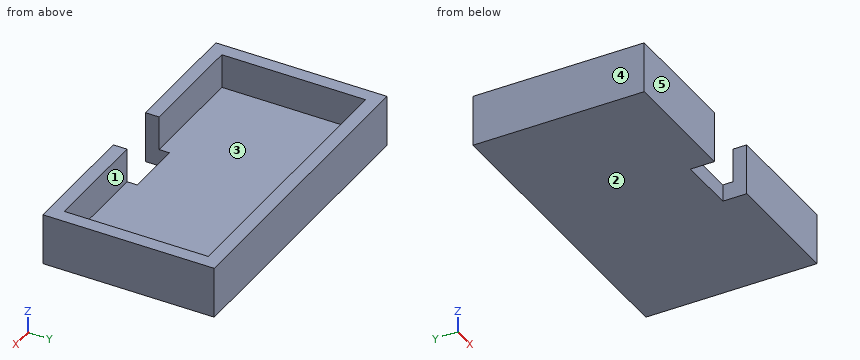
```python
from build123d import *

# Parameters (mm, degrees)
F0_W     = 57.15
F0_H     = 31.75
F1_DEPTH = 9.525
F2_W     = 52.07
F2_H     = 26.67
F3_DEPTH = 6.35
F4_W     = 10.668
F4_H     = 2.54
F4_H_2   = 1.905
F5_DEPTH = 25.4


with BuildPart() as f1:
    # F0 (on Top) → F1 (new body)
    with BuildSketch(Plane.XY):
        Rectangle(F0_W, F0_H)
    extrude(amount=F1_DEPTH)

    # F2 (on face) → F3 (cut)
    with BuildSketch(Plane.XY.offset(9.525)):
        Rectangle(F2_W, F2_H)
    extrude(amount=-F3_DEPTH, mode=Mode.SUBTRACT)

    # F4 (on face) → F5 (cut)
    with BuildSketch(Plane.XY.offset(9.525)):
        with Locations((0, -14.605)):
            Rectangle(F4_W, F4_H)
        with Locations((0, -12.3825)):
            Rectangle(F4_W, F4_H_2)
    extrude(amount=-F5_DEPTH, mode=Mode.SUBTRACT)


solid = f1.part
```
Can you work these out from the model? Positions are in its coordinate system, mm. Face numbers are marked on the shaded views. A direction names the side the tool comes from. Coordinates: 2 decimals unless noted, no trailing zeros. Loops run counter-clockwise (first coordinate to the right, second up) from the corner with the lowest first, then second, coordinate; pieces in that order, holes last.
Item 1: Which directions (+Z, -Z, +X, -X, +Y, -Y) give clear straight access to the entire face, cutting with the end or side of a thin tool? Please do the marked faces 1 and 2.
Answers below:
face 1: +Z
face 2: -Z, +X, -X, +Y, -Y
Item 2: If we mould it in two halves opening along X, with no side actions, what happens to the marked faces 3, 4 and 5? For each: released by +X, released by -X, zero draft, split by the parting line, or undercut.
Answers below:
face 3: undercut
face 4: released by -X
face 5: zero draft
Item 3: Suppose I cut it at B-B (x = -10). Please give me the cut outline in (y, z) (3 decimals).
Answers below:
outline: (-15.875, 0) - (15.875, 0) - (15.875, 9.525) - (13.335, 9.525) - (13.335, 3.175) - (-13.335, 3.175) - (-13.335, 9.525) - (-15.875, 9.525) - close
Item 4: Suppose I cut it at A-A (z = 7.75). Please give me the cut outline in (x, y) (3 decimals), then the cut area to 3 significant figures.
Answers below:
outline: (-28.575, -15.875) - (-5.334, -15.875) - (-5.334, -13.335) - (-26.035, -13.335) - (-26.035, 13.335) - (26.035, 13.335) - (26.035, -13.335) - (5.334, -13.335) - (5.334, -15.875) - (28.575, -15.875) - (28.575, 15.875) - (-28.575, 15.875) - close
area: 399 mm2
Item 5: Suppose I cut it at C-C (y = -8). Please give me the cut outline in (x, z) (3 decimals).
Answers below:
outline: (-28.575, 0) - (28.575, 0) - (28.575, 9.525) - (26.035, 9.525) - (26.035, 3.175) - (-26.035, 3.175) - (-26.035, 9.525) - (-28.575, 9.525) - close
Item 6: Please list where these lines run through material, in increasing order: L1, parallel to Y at x = 11, z = 5.75 (3 decimals); L2, parallel to X at y = -14, z = 4.5 (3 decimals); L3, parallel to X at y = -5, z = 7.75 (3 decimals).
Answers below:
L1: y = -15.875 to -13.335, 13.335 to 15.875
L2: x = -28.575 to -5.334, 5.334 to 28.575
L3: x = -28.575 to -26.035, 26.035 to 28.575
Item 7: I'm going to push flat-ended pins straight in: pin 1 (3 mm diameter, centred on x = 16, y = 4, fed in from -Z); pin 2 (1 mm diameter, centred on x = 1.5, z = 1, fed in from -Y); pin 3 (3 mm diameter, centred on x = 1, y = -6.5, fed in from +Z) (3 decimals). Where does each tip first touch, or does it pass through?
Answers below:
pin 1: stops at z = 0
pin 2: stops at y = -11.43
pin 3: stops at z = 3.175
